The model under review builds one solid part; all positions refer to its coordinate system, in mm. A direction names the side the tool comes from. Round coordinates to 2 decimals unless told otherwise and drop trailing zeros. Write each loop counter-clockwise with the first axis right and the second up, starting at its lowest first coordinate (ties: lowest second). Pieces come first, ordered by that corner, then holes. Notation, with made-up numbers: M 17.25,-29 L 39.25,-29 A23 ccw 39.25,-6 Z; hole C 69.5,3 d7. An arc over 180 degrees is marked long. Write item = value, one per line. Start each with the question number.
Item 1: Take a section at D-D, the plane x = 5.75. Give the boundary of the cut face in (y, z).
Item 2: For pin 1 Ø1 at (y, z) = (7, 2.5) entering from +X; pin 2 Ø3 at (x, y) = (2, 2) entering from -Z; pin 3 Ø8 at (x, y) = (6.5, 1.5) entering from +Z, all flat-tipped, find the tip position at first contact; note any pin that passes through.
Item 3: To check wall thickness, follow line 1 along Z through (x, y) = (0, 10.5); line 2 along Y through (x, z) = (-1.25, 7.5). State the ranges of each line that lie inside material, in increasing order.
Item 4: Take a section at A-A, the plane z = 0. Give the boundary of the cut face in (x, y).
Item 5: Tool access review of faces 1 (the flat face through (-2, 1.5, -6)), 2 (the flat face through (2, 14.2, 2)): name each direction out of +Z, -Z, +X, -X, +Y, -Y from which nothing blocks a thin tool from reaching the whole face with its end or side.
Item 6: The part is to be moulded in two halves that separate along Z. For faces 3 (the cylindrical face through (1.172, 0.74, -8.923)), 4 (the flat face through (-2, 0, -2)), 5 (the cylindrical face through (0, 7, 2)), say which applies: +Z half, -Z half, draft (parallel to the pull), parting line (faces both ways), or undercut.
Item 7: Take a section at C-C, the plane y = 6.5. Give the boundary of the cut face in (x, z), plus the area to 3 significant figures.
Item 8: Take a section at B-B, the plane x = 0. Give the boundary of the cut face in (y, z).
Autodesk Inventor part; units mm, degrees
ref_plane "YZ Plane" through (0, 0, 0) normal (1, 0, 0) x (0, 1, 0)
ref_plane "XZ Plane" through (0, 0, 0) normal (0, 1, 0) x (-1, 0, 0)
ref_plane "XY Plane" through (0, 0, 0) normal (0, 0, 1) x (1, 0, 0)
sketch "Sketch1" plane through (0, 0, 0) normal (0, 1, 0) x (-1, 0, 0)
  circle A0 centre (0, 0) radius 9
  dimension "d0" = 18
extrude "Extrusion1" add sketch "Sketch1" along normal blind 1.5
sketch "Sketch2" plane through (0, 1.5, 0) normal (0, 1, 0) x (1, 0, 0)
  circle A0 centre (0, 0) radius 6.05
  dimension "d3" = 12.1
extrude "Extrusion2" add sketch "Sketch2" along normal blind 11.2
sketch "Sketch3" plane through (0, 12.7, 0) normal (0, 1, 0) x (1, 0, 0)
  circle A0 centre (0, 0) radius 9
  dimension "d6" = 18
extrude "Extrusion3" add sketch "Sketch3" along normal blind 1.5
sketch "Sketch4" plane through (0, 14.2, 0) normal (0, 1, 0) x (1, 0, 0)
  circle A0 centre (0, 0) radius 6.05
  circle A1 centre (0, 0) radius 2
  dimension "d9" = 4
extrude "Extrusion4" cut sketch "Sketch4" against normal through all contours A1
properties part number "10mm_Idle_Pulley_3M"
Response values:
q1.outline = M 0,-6.92 L 1.5,-6.92 L 1.5,-1.88 L 12.7,-1.88 L 12.7,-6.92 L 14.2,-6.92 L 14.2,6.92 L 12.7,6.92 L 12.7,1.88 L 1.5,1.88 L 1.5,6.92 L 0,6.92 Z
q2.pin_1 = 5.71
q2.pin_2 = -8.98
q2.pin_3 = 8.65
q3.line_1 = -6.05 to -2, 2 to 6.05
q3.line_2 = 0 to 1.5, 12.7 to 14.2
q4.outline = M -9,0 L -2,0 L -2,14.2 L -9,14.2 L -9,12.7 L -6.05,12.7 L -6.05,1.5 L -9,1.5 Z; M 2,0 L 9,0 L 9,1.5 L 6.05,1.5 L 6.05,12.7 L 9,12.7 L 9,14.2 L 2,14.2 Z
q5.face_1 = none
q5.face_2 = +Z, -Z, +X, -X, +Y
q6.face_3 = parting line
q6.face_4 = draft
q6.face_5 = undercut
q7.outline = C 0,0 d12.1; hole C 0,0 d4
q7.area = 102 mm2
q8.outline = M 0,-9 L 1.5,-9 L 1.5,-6.05 L 12.7,-6.05 L 12.7,-9 L 14.2,-9 L 14.2,-2 L 0,-2 Z; M 0,2 L 14.2,2 L 14.2,9 L 12.7,9 L 12.7,6.05 L 1.5,6.05 L 1.5,9 L 0,9 Z
